```python
from build123d import *

# Parameters (mm, degrees)
SKETCH_1_W          = 39.9
SKETCH_1_H          = 20
EXTRUDE_1_DEPTH     = 5
SKETCH_2_R          = 1.5
CUT_EXTRUDE_1_DEPTH = 5
SKETCH_4_W          = 39.9
SKETCH_4_H          = 5
EXTRUDE_2_DEPTH     = 45


with BuildPart() as part:
    # 草图1 → 凸台-拉伸1 (new body)
    with BuildSketch(Plane(origin=(0, 0, 0), x_dir=(1, 0, 0), z_dir=(0, 1, 0))):
        with Locations((-19.95, 10)):
            Rectangle(SKETCH_1_W, SKETCH_1_H)
    extrude(amount=EXTRUDE_1_DEPTH)

    # 草图2 → 切除-拉伸1 (cut)
    with BuildSketch(Plane(origin=(0, 5, 0), x_dir=(1, 0, 0), z_dir=(0, 1, 0))):
        with Locations(Location((-27.95, 17.5, 0), (0, 0, 270))):
            Circle(SKETCH_2_R)
        with Locations(Location((-11.95, 17.5, 0), (0, 0, 270))):
            Circle(SKETCH_2_R)
        with Locations(Location((-11.95, 2.5, 0), (0, 0, 90))):
            Circle(SKETCH_2_R)
        with Locations(Location((-27.95, 2.5, 0), (0, 0, 90))):
            Circle(SKETCH_2_R)
    extrude(amount=-CUT_EXTRUDE_1_DEPTH, mode=Mode.SUBTRACT)

    # 草图4 → 凸台-拉伸2 (add)
    with BuildSketch(Plane.XY):
        with Locations((-19.95, 2.5)):
            Rectangle(SKETCH_4_W, SKETCH_4_H)
    extrude(amount=EXTRUDE_2_DEPTH)


solid = part.part
```
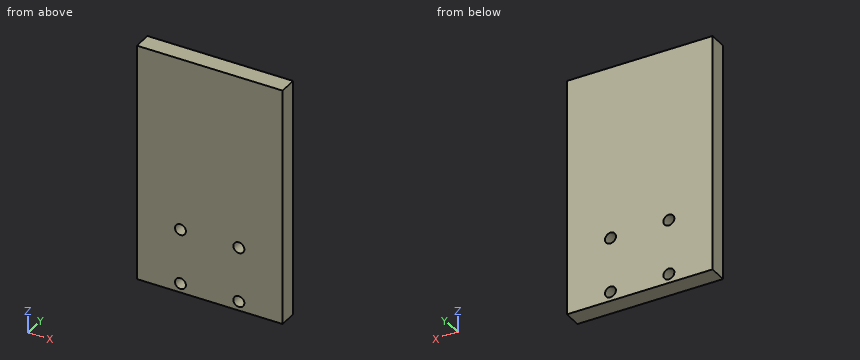
Geometry check sheet. Reference: the model listing, model coordinates, mm. Round coordinates to 2 decimals unless told otherwise and drop trailing zeros. Write each loop counter-clockwise with the first axis right and the second up, starting at its lowest first coordinate (ties: lowest second). Pieces come first, ordered by that corner, then holes. Notation, with made-up numbers: (-31, 62) -> (3, 62) arc R26 ccw to (3, 78) -> close; hole circle Ø3 at (19.25, 10.5). An arc over 180 degrees is marked (long way). Put each result on its own line as item: value.
1) Depth check by flat-ended pin: P1, Ø5, axis at x = -27.95, z = -17.5, coming from the -Y side; P2, Ø1.8, axis at x = -11.95, z = -17.5, coming from the +Y side. Enter the tip coordinate at first touch or a pass-through.
Recorded:
P1: stops at y = 0
P2: passes through
2) Cross-section at B-B, the plane x = -27.95. Enter the section's corners in (y, z).
Recorded:
outline: (0, -20) -> (5, -20) -> (5, -19) -> (0, -19) -> close; (0, -16) -> (5, -16) -> (5, -4) -> (0, -4) -> close; (0, -1) -> (5, -1) -> (5, 45) -> (0, 45) -> close
3) Thickness scan on probe 1 along X at (y, z) = (1.8, -2.5). Record the ranges inside material, lowest first. Write a range as from..to.
Recorded:
probe 1: x = -39.9..-29.45, -26.45..-13.45, -10.45..0
4) Cross-section at A-A, the plane z = -17.5. Enter the section's corners in (x, y).
Recorded:
outline: (-39.9, 0) -> (-29.45, 0) -> (-29.45, 5) -> (-39.9, 5) -> close; (-26.45, 0) -> (-13.45, 0) -> (-13.45, 5) -> (-26.45, 5) -> close; (-10.45, 0) -> (0, 0) -> (0, 5) -> (-10.45, 5) -> close
